Part model, mm, in its own coordinate system. Face numbers are marked on the shaded views. A direction names the side the tool comes from. Coordinates: 2 decimals unless noted, no trailing zeros. Order: outer loops, then holes, each group sorted by start corner. A loop starts at its lowest first (then second) coordinate and runs counter-clockwise, first axis right, second up.
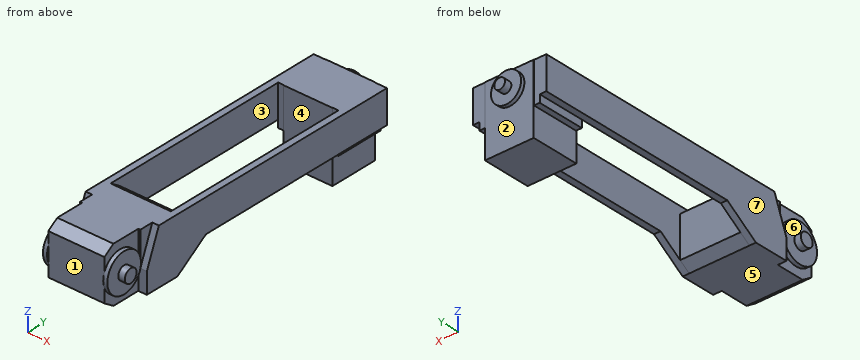
from build123d import *
from OCP.BRepFilletAPI import BRepFilletAPI_MakeChamfer

# Parameters (mm, degrees)
SKETCH1_W           = 41
SKETCH1_H           = 40.2
BOSS_EXTRUDE1_DEPTH = 61.1
SKETCH2_R           = 14
BOSS_EXTRUDE2_DEPTH = 3
SKETCH3_R           = 4.9
BOSS_EXTRUDE3_DEPTH = 4.8
CHAMFER1_SIZE       = 7.5
CHAMFER1_SIZE2      = 5.1
MIRROR5_START       = -20.5
MIRROR5_DEPTH       = 41
BOSS_EXTRUDE4_DEPTH = 1.5
BOSS_EXTRUDE5_DEPTH = 4.7625
SKETCH7_W           = 35.6
SKETCH7_H           = 50.6
BOSS_EXTRUDE6_DEPTH = 35.5
SKETCH9_W           = 29.5
SKETCH9_H           = 35
BOSS_EXTRUDE7_DEPTH = 39.8
SKETCH10_R          = 11
BOSS_EXTRUDE8_DEPTH = 2.75
SKETCH11_R          = 3.9
BOSS_EXTRUDE9_DEPTH = 5.35


# Read off the part's stored shape, not the designer's step: Mirror5
with BuildPart() as part:
    # Sketch1 → Boss-Extrude1 (new body)
    with BuildSketch(Plane(origin=(0, -13, 0), x_dir=(-1, 0, 0), z_dir=(0, 1, 0))):
        Rectangle(SKETCH1_W, SKETCH1_H)
    extrude(amount=BOSS_EXTRUDE1_DEPTH)

    # Sketch2 → Boss-Extrude2 (add)
    with BuildSketch(Plane.ZY.offset(20.5)):
        with Locations(Location((0, 0, 0), (0, 0, 248.213210702))):
            Circle(SKETCH2_R)
    boss_extrude2 = extrude(amount=BOSS_EXTRUDE2_DEPTH)

    # Sketch3 → Boss-Extrude3 (add)
    with BuildSketch(Plane.ZY.offset(23.5)):
        Circle(SKETCH3_R)
    boss_extrude3 = extrude(amount=BOSS_EXTRUDE3_DEPTH)

    # Chamfer1: one chamfer whose edges measure the first distance from different faces: ONE call of the kernel's chamfer builder (chamfer() names one face for all edges)
    chamfer1_edges_1 = [part.edges().sort_by_distance(p)[0] for p in [
        (0, 48.1, -20.1),
    ]]
    chamfer1_side_1 = [part.faces().sort_by_distance(p)[0] for p in [
        (0, 17.55, -20.1),
    ]]
    chamfer1_edges_2 = [part.edges().sort_by_distance(p)[0] for p in [
        (0, 48.1, 20.1),
    ]]
    chamfer1_side_2 = [part.faces().sort_by_distance(p)[0] for p in [
        (0, 17.55, 20.1),
    ]]
    chamfer1 = BRepFilletAPI_MakeChamfer(part.part.solid().wrapped)
    for e in chamfer1_edges_1:
        chamfer1.Add(CHAMFER1_SIZE, CHAMFER1_SIZE2, e.wrapped, chamfer1_side_1[0].wrapped)  # the first distance lies on this face
    for e in chamfer1_edges_2:
        chamfer1.Add(CHAMFER1_SIZE, CHAMFER1_SIZE2, e.wrapped, chamfer1_side_2[0].wrapped)  # the first distance lies on this face
    add(Compound.cast(chamfer1.Shape()), mode=Mode.REPLACE)

    # Mirror5 outline → Mirror5 (cut)
    with BuildSketch(Plane.YZ.offset(MIRROR5_START)):
        Polygon((-13, 20.1), (-13, 15), (-5.5, 20.1), align=None)
        Polygon((-5.5, -20.1), (-13, -15), (-13, -20.1), align=None)
    extrude(amount=MIRROR5_DEPTH, mode=Mode.SUBTRACT)

    # Sketch4 → Boss-Extrude4 (add)
    with BuildSketch(Plane.ZY.offset(20.5)):
        Polygon((-20.1, 15.2), (20.1, 15.2), (20.1, 40.6), (15, 48.1), (-15, 48.1), (-20.1, 40.6), align=None)
    boss_extrude4 = extrude(amount=BOSS_EXTRUDE4_DEPTH)

    # Mirror1: Boss-Extrude2, Boss-Extrude3, Boss-Extrude4 across plane
    add(boss_extrude2.mirror(Plane(origin=(0, 0, 0), x_dir=(0, 0, 1), z_dir=(1, 0, 0))))
    add(boss_extrude3.mirror(Plane(origin=(0, 0, 0), x_dir=(0, 0, 1), z_dir=(1, 0, 0))))
    add(boss_extrude4.mirror(Plane(origin=(0, 0, 0), x_dir=(0, 0, 1), z_dir=(1, 0, 0))))

    # Sketch6 → Boss-Extrude5 (add)
    with BuildSketch(Plane(origin=(22, 0, 0), x_dir=(0, 0, -1), z_dir=(1, 0, 0))):
        Polygon((20.1, 15.2), (20.1, 40.6), (3.9, 64.423529412), (3.9, 215.2), (-20.1, 215.2), (-20.1, 25.2), (4.9, 15.2), align=None)
    boss_extrude5 = extrude(amount=BOSS_EXTRUDE5_DEPTH)

    # Mirror2: Boss-Extrude5 across plane
    add(boss_extrude5.mirror(Plane(origin=(0, 0, 0), x_dir=(0, 0, 1), z_dir=(1, 0, 0))))



with BuildPart() as body_2:
    # Sketch7 → Boss-Extrude6 (new body)
    with BuildSketch(Plane(origin=(0, 215.45, 0), x_dir=(-1, 0, 0), z_dir=(0, 1, 0))):
        with Locations((0, -5.2)):
            Rectangle(SKETCH7_W, SKETCH7_H)
    extrude(amount=-BOSS_EXTRUDE6_DEPTH)


with BuildPart() as part_1:
    add(part.part)

    add(body_2.part)  # Boss-Extrude7 merges body 2
    # Sketch9 → Boss-Extrude7 (add)
    with BuildSketch(Plane.ZY.offset(-22)):
        with Locations((5.35, 197.7)):
            Rectangle(SKETCH9_W, SKETCH9_H)
    boss_extrude7 = extrude(amount=BOSS_EXTRUDE7_DEPTH)

    # Mirror3: Boss-Extrude7 across plane
    add(boss_extrude7.mirror(Plane(origin=(0, 0, 0), x_dir=(0, 0, 1), z_dir=(1, 0, 0))))

    # Sketch10 → Boss-Extrude8 (add)
    with BuildSketch(Plane(origin=(0, 215.45, 0), x_dir=(-1, 0, 0), z_dir=(0, 1, 0))):
        with Locations(Location((0, 8.1, 0), (0, 0, 270))):
            Circle(SKETCH10_R)
    extrude(amount=BOSS_EXTRUDE8_DEPTH)

    # Sketch11 → Boss-Extrude9 (add)
    with BuildSketch(Plane(origin=(0, 218.2, 0), x_dir=(-1, 0, 0), z_dir=(0, 1, 0))):
        with Locations(Location((0, 8.1, 0), (0, 0, 90))):
            Circle(SKETCH11_R)
    extrude(amount=BOSS_EXTRUDE9_DEPTH)


solid = part_1.part
Q1. Which spindle directions (+Z, -Z, +X, -X, +Y, -Y) get a long thin tool onto all of the face, cutting with end or side? Do the marked faces 4, 5, 6 and 7. Say none if no direction does.
Results list:
face 4: +Z, -Z
face 5: -Z, +X, -X, -Y
face 6: -X
face 7: +Z, -Z, -X, +Y
Q2. Cut at B-B on x = 0. Write the cut outline in (y, z), and give its area (3 significant figures).
Results list:
outline: (-13, -15) - (-5.5, -20.1) - (40.6, -20.1) - (48.1, -15) - (48.1, 15) - (40.6, 20.1) - (-5.5, 20.1) - (-13, 15) - close; (179.95, -30.5) - (215.45, -30.5) - (215.45, -2.9) - (218.2, -2.9) - (218.2, 4.2) - (223.55, 4.2) - (223.55, 12) - (218.2, 12) - (218.2, 19.1) - (215.45, 19.1) - (215.45, 20.1) - (179.95, 20.1) - close
area: 4,280 mm2
Q3. Cut at D-D on y = 0. Write the cut outline in (x, z), and give its area (3 significant figures).
Results list:
outline: (-28.3, -4.9) - (-23.5, -4.9) - (-23.5, -14) - (-20.5, -14) - (-20.5, -20.1) - (20.5, -20.1) - (20.5, -14) - (23.5, -14) - (23.5, -4.9) - (28.3, -4.9) - (28.3, 4.9) - (23.5, 4.9) - (23.5, 14) - (20.5, 14) - (20.5, 20.1) - (-20.5, 20.1) - (-20.5, 14) - (-23.5, 14) - (-23.5, 4.9) - (-28.3, 4.9) - close
area: 1,910 mm2
Q4. Cut at C-C on z = -18. Write the cut outline in (x, y).
Results list:
outline: (-26.76, 15.2) - (-20.5, 15.2) - (-20.5, -8.59) - (20.5, -8.59) - (20.5, 15.2) - (26.76, 15.2) - (26.76, 43.69) - (-26.76, 43.69) - close; (-17.8, 179.95) - (17.8, 179.95) - (17.8, 215.45) - (-17.8, 215.45) - close
Q5. Cut at A-A on y = 118. Write the cut outline in (x, z).
Results list:
outline: (-26.76, -3.9) - (-22, -3.9) - (-22, 20.1) - (-26.76, 20.1) - close; (22, -3.9) - (26.76, -3.9) - (26.76, 20.1) - (22, 20.1) - close
Q6. Mould opens along Y. For the marked faces 1, 2 and 3 say: pulls with the +Y half, pulls with the -Y half, needs draft (parallel to the pull), parting line crosses it, or undercut.
Results list:
face 1: pulls with the -Y half
face 2: pulls with the +Y half
face 3: undercut
Q7. Wall check: line 1 along X through (y, z) = (128, 14); line 2 along Y through (x, z) = (-10, -12); line 3 along X through (y, z) = (202, -7). Give the ranges that are in metal, low to high.
Results list:
line 1: x = -26.76 to -22, 22 to 26.76
line 2: y = -13 to 48.1, 179.95 to 215.45
line 3: x = -22 to 22
Q8. Pin check, flat tips, straight feed: pin 1 Ø1.9 at (x, z) = (24, -4) entering from -Y; pin 2 Ø2 at (y, z) = (57, -4) entering from -X; pin 3 Ø0.8 at (y, z) = (-13.5, 0.5) entering from -X. Stop position of each tip, or through.
Results list:
pin 1: stops at y = -13.63
pin 2: stops at x = -26.76
pin 3: stops at x = -23.5
